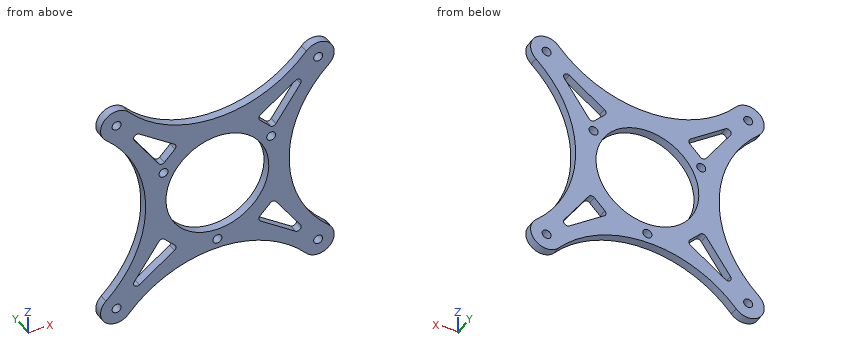
from build123d import *

# Parameters (mm, degrees)
SKETCH_1_R          = 2.1
SKETCH_1_R_2        = 15
EXTRUDE_1_DEPTH     = 4
SKETCH_3_R          = 24
CUT_EXTRUDE_2_DEPTH = 78.210284473
CUT_EXTRUDE_3_DEPTH = 78.210284473
FILLET_1_R          = 1.7


with BuildPart() as part:
    # 草图1 → 凸台-拉伸1 (new body)
    with BuildSketch(Plane(origin=(0, 0, 0), x_dir=(1, 0, 0), z_dir=(0, 1, 0))):
        with BuildLine():
            ThreePointArc((-41.42868058, 52.018404679), (-52.325901808, 52.325901808), (-52.018404679, 41.42868058))
            ThreePointArc((-52.018404679, 41.42868058), (-33.472279505, 0), (-52.018404679, -41.42868058))
            ThreePointArc((-52.018404679, -41.42868058), (-52.325901808, -52.325901808), (-41.42868058, -52.018404679))
            ThreePointArc((-41.42868058, -52.018404679), (0, -33.472279505), (41.42868058, -52.018404679))
            ThreePointArc((41.42868058, -52.018404679), (52.325901808, -52.325901808), (52.018404679, -41.42868058))
            ThreePointArc((52.018404679, -41.42868058), (33.472279505, 0), (52.018404679, 41.42868058))
            ThreePointArc((52.018404679, 41.42868058), (52.325901808, 52.325901808), (41.42868058, 52.018404679))
            ThreePointArc((41.42868058, 52.018404679), (0, 33.472279505), (-41.42868058, 52.018404679))
        make_face()
        with Locations(Location((0, 29, 0), (0, 0, 270))):
            Circle(SKETCH_1_R, mode=Mode.SUBTRACT)
        with Locations(Location((25.11473671, -14.5, 0), (0, 0, 270))):
            Circle(SKETCH_1_R, mode=Mode.SUBTRACT)
        with Locations(Location((-25.11473671, -14.5, 0), (0, 0, 270))):
            Circle(SKETCH_1_R, mode=Mode.SUBTRACT)
        with Locations(Location((47.022600949, 47.022600949, 0), (0, 0, 270))):
            Circle(SKETCH_1_R, mode=Mode.SUBTRACT)
        with Locations(Location((47.022600949, -47.022600949, 0), (0, 0, 90))):
            Circle(SKETCH_1_R, mode=Mode.SUBTRACT)
        with Locations(Location((-47.022600949, -47.022600949, 0), (0, 0, 270))):
            Circle(SKETCH_1_R, mode=Mode.SUBTRACT)
        with Locations(Location((-47.022600949, 47.022600949, 0), (0, 0, 90))):
            Circle(SKETCH_1_R, mode=Mode.SUBTRACT)
        with Locations(Location((0, 0, 0), (0, 0, 270))):
            Circle(SKETCH_1_R_2, mode=Mode.SUBTRACT)
    extrude(amount=EXTRUDE_1_DEPTH)

    # 草图3 → 切除-拉伸2 (cut, through all)
    with BuildSketch(Plane.XZ):
        with Locations(Location((0, 0, 0), (0, 0, 270))):
            Circle(SKETCH_3_R)
    extrude(amount=-CUT_EXTRUDE_2_DEPTH, mode=Mode.SUBTRACT)

    # 草图4 → 切除-拉伸3 (cut, through all)
    with BuildSketch(Plane.XZ):
        Polygon((-44.329973687, 44.329973687), (-26.162950904, 18.384776311), (-18.384776311, 26.162950904), align=None)
        Polygon((26.162950904, 18.384776311), (44.329973687, 44.329973687), (18.384776311, 26.162950904), align=None)
        Polygon((18.384776311, -26.162950904), (44.329973687, -44.329973687), (26.162950904, -18.384776311), align=None)
        Polygon((-26.162950904, -18.384776311), (-44.329973687, -44.329973687), (-18.384776311, -26.162950904), align=None)
    extrude(amount=-CUT_EXTRUDE_3_DEPTH, mode=Mode.SUBTRACT)

    # 圆角1
    fillet_1_edges = [part.edges().sort_by_distance(p)[0] for p in [
        (-18.384776311, 2, -26.162950904),
        (-44.329973687, 2, -44.329973687),
        (-26.162950904, 2, -18.384776311),
        (26.162950904, 2, -18.384776311),
        (44.329973687, 2, -44.329973687),
        (18.384776311, 2, -26.162950904),
        (18.384776311, 2, 26.162950904),
        (44.329973687, 2, 44.329973687),
        (26.162950904, 2, 18.384776311),
        (-44.329973687, 2, 44.329973687),
        (-18.384776311, 2, 26.162950904),
        (-26.162950904, 2, 18.384776311),
    ]]
    fillet(fillet_1_edges, radius=FILLET_1_R)


solid = part.part
Source: CAD feature listing. Evaluate the final solid. Frame: model axes, mm. Coordinates: 2 decimals unless noted, no trailing zeros. Order: outer loops, then holes, each group sorted by start corner. A loop starts at its lowest first (then second) coordinate and runs counter-clockwise, first axis right, second up.
Item 1: Cut plane C-C (x = -15.5). Return loops of the section in (y, z), plus the area to 3 significant figures.
Output values:
outline: (0, -35.68) - (4, -35.68) - (4, -18.32) - (0, -18.32) - close; (0, 18.32) - (4, 18.32) - (4, 35.68) - (0, 35.68) - close
area: 139 mm2
Item 2: Material intervals for line 1 (X direction, y = 3, z = -26); line 2 (Z direction, x = -29, y = 0.5); line 3 (X direction, y = 1.7, z = 14.5), sorted ascending.
Output values:
line 1: x = -39.93 to -31.5, -19.32 to 19.32, 31.5 to 39.93
line 2: z = -41.64 to -33.6, -22.44 to 22.44, 33.6 to 41.64
line 3: x = -35.4 to -27.21, -23.01 to -19.12, 19.12 to 23.01, 27.21 to 35.4
Item 3: Cut plane D-D (z = 30). Return loops of the section in (x, y), plus the area to 3 significant figures.
Output values:
outline: (-42.27, 0) - (-34.3, 0) - (-34.3, 4) - (-42.27, 4) - close; (-23.86, 0) - (23.86, 0) - (23.86, 4) - (-23.86, 4) - close; (34.3, 0) - (42.27, 0) - (42.27, 4) - (34.3, 4) - close
area: 255 mm2
Item 4: First-contact query: P1, Ø1, axis at x = -6, y = 2, coming from the +Z side. Flat tip, straight axial feed; report the tip coordinate or a pass-through.
Output values:
P1: stops at z = 33.85
Item 5: Cut plane A-A (x = 0). Return loops of the section in (y, z).
Output values:
outline: (0, -33.47) - (4, -33.47) - (4, -31.1) - (0, -31.1) - close; (0, -26.9) - (4, -26.9) - (4, -24) - (0, -24) - close; (0, 24) - (4, 24) - (4, 33.47) - (0, 33.47) - close
Item 6: Cut plane B-B (z = 0). Return loops of the section in (x, y), plus the area to 3 significant figures.
Output values:
outline: (-33.47, 0) - (-24, 0) - (-24, 4) - (-33.47, 4) - close; (24, 0) - (33.47, 0) - (33.47, 4) - (24, 4) - close
area: 75.8 mm2
